```python
from build123d import *

# Parameters (mm, degrees)
F0_R     = 16.85
F1_DEPTH = 25
F2_R     = 22.410556
F2_R_2   = 15.4
F3_DEPTH = 15
F4_R     = 22.657316
F4_R_2   = 15.4
F5_DEPTH = 5


with BuildPart() as f1:
    # F0 (on Front) → F1 (new body)
    with BuildSketch(Plane.XZ):
        Circle(F0_R)
    extrude(amount=-F1_DEPTH)

    # F2 (on Front) → F3 (cut)
    with BuildSketch(Plane.XZ):
        Circle(F2_R)
        Circle(F2_R_2, mode=Mode.SUBTRACT)
    extrude(amount=-F3_DEPTH, mode=Mode.SUBTRACT)

    # F4 (on face) → F5 (cut)
    with BuildSketch(Plane(origin=(0, 25, 0), x_dir=(-1, 0, 0), z_dir=(0, 1, 0))):
        Circle(F4_R)
        Circle(F4_R_2, mode=Mode.SUBTRACT)
    extrude(amount=-F5_DEPTH, mode=Mode.SUBTRACT)


solid = f1.part
```
Verification items for the finished model (mm, model axes). A direction names the side the tool comes from. Coordinates: 2 decimals unless noted, no trailing zeros. Write each loop counter-clockwise with the first axis right and the second up, starting at its lowest first coordinate (ties: lowest second). Pieces come first, ordered by that corner, then holes. Notation, with made-up numbers: (17, -1) - (50, -1) arc R21 ccw to (50, 6) - close; hole circle Ø1 at (-21.5, 85). An arc over 180 degrees is marked (long way). One line per question, with ' | ' between items. Start each with the question number.
1. Material ranges on line 1 along X through (y, z) = (9, 0.5); line 2 along Y through (x, z) = (6.5, 15); line 3 along Z through (x, y) = (12.5, 16), recorded low to high.
2. Section check A-A (x = 0). Enter the section's corners in (y, z), plus the area to 4 significant figures.
3. Gauge pin test, flat ends, axial feed: P1, Ø8, axis at x = -11.5, y = 16.5, coming from the +Z side; P2, Ø1.5, axis at x = -2, y = 12.5, coming from the -Z side; P3, Ø5, axis at x = -3, y = 17.5, coming from the -Z side; P4, Ø17, axis at x = 1.5, z = -3.5, coming from the -Y side. Record the tip position at first contact, or that the pin passes through.
4. Section check C-C (y = 22.5). Enter the section's corners in (x, z), plus the area to 3 significant figures.
5. Section check B-B (z = 0). Enter the section's corners in (x, y).
6. Access from +Z, -Z, +X, -X, +Y, -Y to the whole of each face (thin tool, end or side, straight path). Record for faces 1 (the cylindrical face through (3.338, 22.535, -15.034)), 2 (the cylindrical face through (-3.338, 7.395, -15.034)), 3 (the flat face through (0, 25, 0)).
Computed values:
1) line 1: -15.39 to 15.39 | line 2: 15 to 20 | line 3: -11.3 to 11.3
2) outline: (0, -15.4) - (15, -15.4) - (15, -16.85) - (20, -16.85) - (20, -15.4) - (25, -15.4) - (25, 15.4) - (20, 15.4) - (20, 16.85) - (15, 16.85) - (15, 15.4) - (0, 15.4) - close | area: 784.5 mm²
3) P1: z = 15.09 | P2: z = -15.35 | P3: z = -16.84 | P4: y = 0
4) outline: circle Ø30.8 at (0, 0) | area: 745 mm²
5) outline: (-16.85, 15) - (-15.4, 15) - (-15.4, 0) - (15.4, 0) - (15.4, 15) - (16.85, 15) - (16.85, 20) - (15.4, 20) - (15.4, 25) - (-15.4, 25) - (-15.4, 20) - (-16.85, 20) - close
6) face 1: +Y | face 2: -Y | face 3: +Z, -Z, +X, -X, +Y
